```python
from build123d import *

# Parameters (mm, degrees)
SKETCH1_W           = 93
SKETCH1_H           = 89
BOSS_EXTRUDE1_DEPTH = 1
SKETCH2_R           = 3
BOSS_EXTRUDE2_DEPTH = 9
SKETCH3_R           = 6.5
SKETCH3_W           = 70
SKETCH3_H           = 10
CUT_EXTRUDE4_DEPTH  = 1
SKETCH4_R           = 2
CUT_EXTRUDE5_DEPTH  = 10


with BuildPart() as part:
    # Sketch1 → Boss-Extrude1 (new body)
    with BuildSketch(Plane(origin=(0, 0, 0), x_dir=(1, 0, 0), z_dir=(0, 1, 0))):
        Rectangle(SKETCH1_W, SKETCH1_H)
    extrude(amount=BOSS_EXTRUDE1_DEPTH)

    # Sketch2 → Boss-Extrude2 (add)
    with BuildSketch(Plane(origin=(0, 1, 0), x_dir=(1, 0, 0), z_dir=(0, 1, 0))):
        with Locations((-43.5, 40.5)):
            Circle(SKETCH2_R)
        with Locations((43.5, 40.5)):
            Circle(SKETCH2_R)
        with Locations((-43.5, -24.5)):
            Circle(SKETCH2_R)
        with Locations((43.5, -24.5)):
            Circle(SKETCH2_R)
    extrude(amount=BOSS_EXTRUDE2_DEPTH)

    # Sketch3 → Cut-Extrude4 (cut)
    with BuildSketch(Plane(origin=(0, 1, 0), x_dir=(1, 0, 0), z_dir=(0, 1, 0))):
        with Locations((-3.5, -35.5)):
            Circle(SKETCH3_R)
        with Locations((0, 39.5)):
            Rectangle(SKETCH3_W, SKETCH3_H)
    extrude(amount=-CUT_EXTRUDE4_DEPTH, mode=Mode.SUBTRACT)

    # Sketch4 → Cut-Extrude5 (cut)
    with BuildSketch(Plane(origin=(0, 10, 0), x_dir=(1, 0, 0), z_dir=(0, 1, 0))):
        with Locations((-43.5, 40.5)):
            Circle(SKETCH4_R)
        with Locations((-43.5, -24.5)):
            Circle(SKETCH4_R)
        with Locations((43.5, 40.5)):
            Circle(SKETCH4_R)
        with Locations((43.5, -24.5)):
            Circle(SKETCH4_R)
    extrude(amount=-CUT_EXTRUDE5_DEPTH, mode=Mode.SUBTRACT)


solid = part.part
```
The model under review builds one solid part; all positions refer to its coordinate system, in mm. A direction names the side the tool comes from. Coordinates: 2 decimals unless noted, no trailing zeros. Order: outer loops, then holes, each group sorted by start corner. A loop starts at its lowest first (then second) coordinate and runs counter-clockwise, first axis right, second up. Notation, with made-up numbers: (19, 78) -> (26, 78) arc R18 cw to (26, 111) -> close; hole circle Ø7 at (39, -21). An arc over 180 degrees is marked (long way). Answer in a Markdown table with one row per item. Add a question column.
Item 1: We need section D-D on x = 43.5. Write out the cut boundary in (y, z).
Item 2: Mouldability with a two-part tool opening along Z and no side actions: class faces 1 (the cylindrical face through (40.5, 5.4, 24.4)), 2 (the flat face through (-44, 10, -43)) as +Z half, -Z half, draft (parallel to the pull), parting line (faces both ways), or undercut.
Item 3: To check wall thickness, follow probe 1 along X at (y, z) = (5.5, 24.5); probe 2 along Z at (x, y) = (-43.5, 2.5); probe 3 along Z at (x, y) = (-3.5, 0.5). State the ranges of each line that lie inside material, in increasing order.
Item 4: Clearance check with flat-ended pins moving along their axes: pin 1 (3 mm diameter, centred on x = 37, y = 3.5, fed in from -Z); pin 2 (0.5 mm diameter, centred on x = -1, y = 0.5, fed in from -Z); pin 3 (4 mm diameter, centred on x = 20.5, z = 23.5, fed in from +Y); pin 4 (5 mm diameter, centred on x = -43.5, z = -40.5, fed in from +Y). State where each tip first meets the part, or that it passes through.
Item 5: Machinability: for faces 3 (the cylindrical face through (-46.5, 5.4, 24.4)), 4 (the flat face through (43, 10, 22)), which of the approach directions +Z, -Z, +X, -X, +Y, -Y give a long, thin tool a straight path to every point of the face, cutting with its end or side? Answer none if there is none.
Item 6: We need section B-B on y = 4. Write out the cut boundary in (x, z), plus the area to 3 significant figures.
Item 7: We need section A-A on z = 35.5. Write out the cut boundary in (x, y).
Item 8: We need section C-C on x = -3.5. Write out the cut boundary in (y, z).
Final values:
| question | item | result |
|---|---|---|
| 1 | outline | (0, -44.5) -> (1, -44.5) -> (1, -43.5) -> (10, -43.5) -> (10, -42.5) -> (0, -42.5) -> close; (0, -38.5) -> (10, -38.5) -> (10, -37.5) -> (1, -37.5) -> (1, 21.5) -> (10, 21.5) -> (10, 22.5) -> (0, 22.5) -> close; (0, 26.5) -> (10, 26.5) -> (10, 27.5) -> (1, 27.5) -> (1, 44.5) -> (0, 44.5) -> close |
| 2 | face 1 | undercut |
| 2 | face 2 | draft |
| 3 | probe 1 | x = -46.5 to -45.5, -41.5 to -40.5, 40.5 to 41.5, 45.5 to 46.5 |
| 3 | probe 2 | z = -43.5 to -42.5, -38.5 to -37.5, 21.5 to 22.5, 26.5 to 27.5 |
| 3 | probe 3 | z = -34.5 to 29, 42 to 44.5 |
| 4 | pin 1 | passes through |
| 4 | pin 2 | stops at z = -34.5 |
| 4 | pin 3 | stops at y = 1 |
| 4 | pin 4 | stops at y = 10 |
| 5 | face 3 | +Y |
| 5 | face 4 | +Z, -Z, +X, -X, +Y |
| 6 | outline | circle Ø6 at (-43.5, -40.5); circle Ø6 at (-43.5, 24.5); circle Ø6 at (43.5, -40.5); circle Ø6 at (43.5, 24.5); hole circle Ø4 at (-43.5, -40.5); hole circle Ø4 at (-43.5, 24.5); hole circle Ø4 at (43.5, -40.5); hole circle Ø4 at (43.5, 24.5) |
| 6 | area | 62.8 mm2 |
| 7 | outline | (-46.5, 0) -> (-10, 0) -> (-10, 1) -> (-46.5, 1) -> close; (3, 0) -> (46.5, 0) -> (46.5, 1) -> (3, 1) -> close |
| 8 | outline | (0, -34.5) -> (1, -34.5) -> (1, 29) -> (0, 29) -> close; (0, 42) -> (1, 42) -> (1, 44.5) -> (0, 44.5) -> close |
